from build123d import *

# Parameters (mm, degrees)
SKETCH_1_W                  = 480
SKETCH_1_H                  = 310
EXTRUDE_1_DEPTH             = 10
SKETCH_2_R                  = 11
CUT_EXTRUDE_1_DEPTH         = 572.489282489
PATTERN_LINEAR_1_COUNT      = 6
PATTERN_LINEAR_1_PITCH      = 80
PATTERN_LINEAR_1_COUNT_DIR2 = 4
PATTERN_LINEAR_1_PITCH_DIR2 = 80


with BuildPart() as part:
    # 草图1 → 拉伸1 (new body)
    with BuildSketch(Plane.XY):
        with Locations((240, 155)):
            Rectangle(SKETCH_1_W, SKETCH_1_H)
    extrude(amount=EXTRUDE_1_DEPTH)

    # 草图2 → 切除-拉伸1 (cut, through all)
    with BuildSketch(Plane.XY.offset(10)):
        with Locations((40, 35)):
            Circle(SKETCH_2_R)
    cut_extrude_1 = extrude(amount=-CUT_EXTRUDE_1_DEPTH, mode=Mode.SUBTRACT)

    # 阵列(线性)1: Cut-Extrude 1 6 × 4
    with Locations(*[(i * PATTERN_LINEAR_1_PITCH, j * PATTERN_LINEAR_1_PITCH_DIR2, 0) for i in range(PATTERN_LINEAR_1_COUNT) for j in range(PATTERN_LINEAR_1_COUNT_DIR2) if (i, j) != (0, 0)]):
        add(cut_extrude_1, mode=Mode.SUBTRACT)


solid = part.part
Part model, mm, in its own coordinate system. Give positions to 0.01 mm unless a question says otherwise; leave off trailing zeros. Loops run counter-clockwise (first coordinate to the right, second up) from the corner with the lowest first, then second, coordinate; pieces in that order, holes last. Notation, with made-up numbers: M 78.25,-7 L 130.25,-7 A23 ccw 130.25,26 Z; hole C 0,-23 d9. An arc over 180 degrees is marked long. Put each result on its own line as item: value. Start each with the question number.
1) Saw through at A-A (x = 440). List the corners of the cut face in (y, z).
2) Saw through at D-D (x = 195.5). List the corners of the cut face in (y, z).
3) Flat gauge pin, fed straight in: pin 1 (20 mm diameter, centred on x = 120, y = 115, fed in from +Z). Where does the tip first touch, or does it go through?
4) Saw through at C-C (z = 7.25). State how many separate pieces and enclosed holes the cut face has, then the cut area to 3 significant figures.
5) Saw through at B-B (y = 275). List the corners of the cut face in (x, z).
6) Probe probe 1 along Y at (x, z) = (360, 7.5); probe 2 along Y at (x, z) = (122, 3.25). List the from-to ranges inside material, lowest first.
7) Pull direction X, two halves, no side cores. Call faces 1 (the cylindrical face through (191.89, 282.43, 5.07)), 2 (the flat face through (237, 157, 10)): +X half, -X half, draft (parallel to the pull), parting line (faces both ways), or undercut.
Numbers:
1. outline: M 0,0 L 24,0 L 24,10 L 0,10 Z; M 46,0 L 104,0 L 104,10 L 46,10 Z; M 126,0 L 184,0 L 184,10 L 126,10 Z; M 206,0 L 264,0 L 264,10 L 206,10 Z; M 286,0 L 310,0 L 310,10 L 286,10 Z
2. outline: M 0,0 L 24.96,0 L 24.96,10 L 0,10 Z; M 45.04,0 L 104.96,0 L 104.96,10 L 45.04,10 Z; M 125.04,0 L 184.96,0 L 184.96,10 L 125.04,10 Z; M 205.04,0 L 264.96,0 L 264.96,10 L 205.04,10 Z; M 285.04,0 L 310,0 L 310,10 L 285.04,10 Z
3. pin 1: through
4. separate pieces: 1
4. enclosed holes: 24
4. area: 140,000 mm^2
5. outline: M 0,0 L 29,0 L 29,10 L 0,10 Z; M 51,0 L 109,0 L 109,10 L 51,10 Z; M 131,0 L 189,0 L 189,10 L 131,10 Z; M 211,0 L 269,0 L 269,10 L 211,10 Z; M 291,0 L 349,0 L 349,10 L 291,10 Z; M 371,0 L 429,0 L 429,10 L 371,10 Z; M 451,0 L 480,0 L 480,10 L 451,10 Z
6. probe 1: 0 to 24, 46 to 104, 126 to 184, 206 to 264, 286 to 310
6. probe 2: 0 to 24.18, 45.82 to 104.18, 125.82 to 184.18, 205.82 to 264.18, 285.82 to 310
7. face 1: undercut
7. face 2: draft
